The model under review builds one solid part; all positions refer to its coordinate system, in mm. Face numbers are marked on the shaded views. A direction names the side the tool comes from. Round coordinates to 2 decimals unless told otherwise and drop trailing zeros. Write each loop counter-clockwise with the first axis right and the second up, starting at its lowest first coordinate (ties: lowest second). Pieces come first, ordered by that corner, then holes.
Item 1: Add section D-D (x = -38). Give the boundary of the cut face in (y, z), plus the area to 3 significant figures.
Item 2: Add section C-C (y = 142). Give the boundary of the cut face in (x, z).
Item 3: To check wall thickness, follow L1, parallel to Y at x = 27, z = -17; L2, parallel to Z at x = -29.5, y = 155.5; L3, parallel to Y at x = -37.5, z = -13. State the ranges of each line that lie inside material, in increasing order.
Item 4: Machinability: for the marked faces 5, 6, 7 and 8, which of the approach directions +Z, -Z, +X, -X, +Y, -Y give a long, thin tool a straight path to every point of the face, cutting with its end or side? Answer none if there is none.
Item 5: Add section B-B (z = -12). Give the boundary of the cut face in (x, y), plus the area to 3 significant figures.
Item 6: Add section A-A (x = 10). Give the boundary of the cut face in (y, z).
Item 7: Clearance check with flat-ended pins moving along their axes: pin 1 Ø10 at (x, y) = (38.5, -73.5) entering from +Z; pin 2 Ø13.5 at (x, y) = (-7.5, 182) entering from -Z; pin 3 Ø3 at (y, z) = (-57, 40) entering from +X. State where each tip first meets the part, or that it passes through.
Item 8: Draft analysis for pull direction Z (two halves, no side actions). For the marked faces 1, 2, 3 and 4, state which applies: +Z half, -Z half, draft (parallel to the pull), parting line (faces both ways), or undercut.
```python
from build123d import *

# Parameters (mm, degrees)
F0_W     = 381
F0_H     = 88.9
F1_DEPTH = 44.45
F4_W     = 12.7
F4_H     = 6.35
F5_DEPTH = 381.001
F6_W     = 88.9
F6_H     = 88.9
F6_W_2   = 38.1
F6_H_2   = 50.8
F7_REACH = 193.287585695
F8_W     = 88.9
F8_H     = 88.9
F8_W_2   = 38.1
F8_H_2   = 50.8
F9_DEPTH = 25.4


with BuildPart() as f1:
    # F0 (on Right) → F1 (new body, symmetric)
    with BuildSketch(Plane.YZ):
        Rectangle(F0_W, F0_H)
    extrude(amount=F1_DEPTH, both=True)

    # F4 (on face) → F5 (cut, through all)
    with BuildSketch(Plane(origin=(0, 190.5, 0), x_dir=(-1, 0, 0), z_dir=(0, 1, 0))):
        with Locations((-38.1, 41.275)):
            Rectangle(F4_W, F4_H)
    extrude(amount=-F5_DEPTH, mode=Mode.SUBTRACT)

    f7_end = Plane(origin=(0, 111.4494145991, 64.3453495198), x_dir=(0, -0.5, 0.8660254038), z_dir=(0, 0.8660254038, 0.5))
    # F6 (on face) → F7 (cut, up to a plane its end follows)
    with BuildSketch(Plane(origin=(0, 190.5, 0), x_dir=(-1, 0, 0), z_dir=(0, 1, 0))):
        Rectangle(F6_W, F6_H)
        Rectangle(F6_W_2, F6_H_2, mode=Mode.SUBTRACT)
    f7_long = extrude(amount=-F7_REACH, mode=Mode.PRIVATE)
    add(split(f7_long, bisect_by=f7_end, keep=Keep.TOP, mode=Mode.PRIVATE), mode=Mode.SUBTRACT)

    # F8 (on face) → F9 (cut)
    with BuildSketch(Plane.XZ.offset(190.5)):
        Rectangle(F8_W, F8_H)
        Rectangle(F8_W_2, F8_H_2, mode=Mode.SUBTRACT)
    extrude(amount=-F9_DEPTH, mode=Mode.SUBTRACT)


solid = f1.part
```
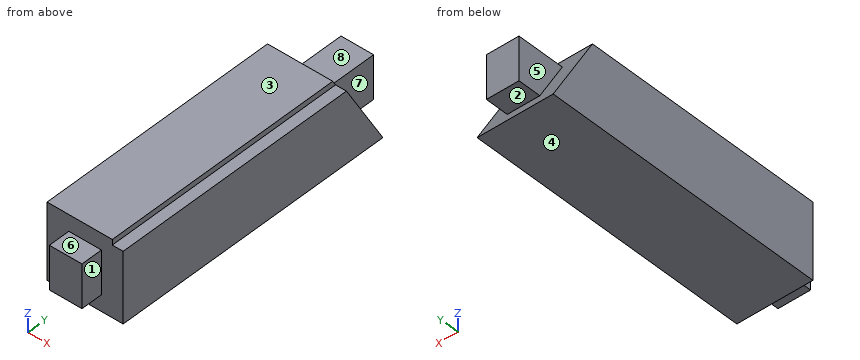
Numbers:
1. outline: (-165.1, -44.45) - (174.26, -44.45) - (122.94, 44.45) - (-165.1, 44.45) - close
1. area: 27,900 mm2
2. outline: (-44.45, -44.45) - (44.45, -44.45) - (44.45, 11.43) - (19.05, 11.43) - (19.05, 25.4) - (-19.05, 25.4) - (-19.05, 11.43) - (-44.45, 11.43) - close
3. L1: y = -165.1 to 158.41
3. L2: z = -44.45 to -11.95
3. L3: y = -165.1 to 156.1
4. face 5: +Z, -X, +Y
4. face 6: +Z, +X, -X, -Y
4. face 7: +Z, +X, +Y
4. face 8: +Z, +X, -X, +Y
5. outline: (-44.45, -165.1) - (-19.05, -165.1) - (-19.05, -190.5) - (19.05, -190.5) - (19.05, -165.1) - (44.45, -165.1) - (44.45, 155.53) - (19.05, 155.53) - (19.05, 190.5) - (-19.05, 190.5) - (-19.05, 155.53) - (-44.45, 155.53) - close
5. area: 30,800 mm2
6. outline: (-190.5, -25.4) - (-165.1, -25.4) - (-165.1, -44.45) - (174.26, -44.45) - (163.26, -25.4) - (190.5, -25.4) - (190.5, 25.4) - (133.93, 25.4) - (122.94, 44.45) - (-165.1, 44.45) - (-165.1, 25.4) - (-190.5, 25.4) - close
7. pin 1: stops at z = 38.1
7. pin 2: stops at z = -25.4
7. pin 3: stops at x = 31.75
8. face 1: draft
8. face 2: undercut
8. face 3: +Z half
8. face 4: -Z half
